Work out the finished part from the listing and answer in its coordinate system (mm). A direction names the side the tool comes from. Give positions to 0.01 mm unless a question says otherwise; leave off trailing zeros. Loops run counter-clockwise (first coordinate to the right, second up) from the corner with the lowest first, then second, coordinate; pieces in that order, holes last. Notation, with made-up numbers: (-8.5, -9.5) - (35.5, -9.5) arc R9 cw to (35.5, 4.5) - close; hole circle Ø1 at (67.25, 87). An arc over 180 degrees is marked (long way). Use one line per item in the form item = value. Start each with the question number.
Solid Edge part; units mm, degrees
sketch "Sketch1" plane through (0, 0, -1.75) normal (0, 0, 1) x (1, 0, 0)
  line L0 (-3.447, 1.4766) -> (7.158, 26.233)
  line L1 (2.2918, -2.9682) -> (23.6093, 13.4911)
  arc A0 (23.6093, 13.4911) -> (7.158, 26.233) centre (17.0395, 22) ccw
  arc A1 (2.2918, -2.9682) -> (-3.447, 1.4766) centre (0, 0) cw
sketch "Sketch2" plane through (17.0395, 0, 0) normal (-1, 0, 0) x (0, -1, 0)
  line L0 (-32.75, -0.3358) -> (-31.3358, -1.75)
  line L1 (-32.75, -3.1642) -> (-31.3358, -1.75)
  line L2 (-32.75, -3.1642) -> (-34.1642, -1.75)
  line L3 (-32.75, -0.3358) -> (-34.1642, -1.75)
sweep "Riemen_Twist" add profiles "Sketch2" path "Sketch1"
properties material "(None)"
1) Find the intervals of material crossed by probe 1 along X at (y, z) = (12, -3); probe 2 along Y at (x, z) = (13, -1.1); probe 3 along Y at (x, z) = (25.5, -1.65), in increasing order.
2) Determine the mould class of faces 4 (the conical face through (23.99, 30.52, -2.92)), 5 (the conical face through (-1.543, -2.07, -1.996)), 6 (the flat face through (13.227, 4.594, -2.467)) for opening direction Y: released by +Y, released by -Y, zero draft, split by the parting line, or undercut.
3) A cutting plane is placed at B-B (z = -2.5). Give the vertices of the cut face in (x, y), plus the area to 3 significant figures.
4) Flat-ended cylindrical pins translate along their axes: pin 1 Ø1 at (x, z) = (16.5, -2) entering from -Y; pin 2 Ø8 at (x, y) = (0.5, 13.5) entering from -Z; pin 3 Ø8 at (x, y) = (8.5, 0) entering from +Z; pin 4 Ø8 at (x, y) = (12.5, 15.5) entering from -Z. Find the tip coordinate at first contact, or state that the pin passes through.
5) A tool of negligible diameter and unlimited length cuts with its end or side. For faces 1 (the flat face through (12.38, 5.7, -1.03)), 2 (the flat face through (2.59, 13.75, -2.45)), 3 (the flat face through (13.24, 4.58, -1.05)), from which of +Z, -Z, +X, -X, +Y, -Y can it reach the whole face along a straight path? Write none if from no direction.
6) A cutting plane is placed at A-A (y = 22). Give the vertices of the cut face in (x, z).
Answer sheet:
q1.probe_1 = 0.88 to 1.24, 21.41 to 21.95
q1.probe_2 = 4.33 to 6.27, 31.13 to 32.78
q1.probe_3 = 13.4 to 17.82, 26.18 to 30.6
q2.face_4 = split by the parting line
q2.face_5 = undercut
q2.face_6 = released by -Y
q3.outline = (-4.06, 1.74) arc R4.41 ccw to (2.7, -3.49) - (24.02, 12.97) arc R11.41 ccw (long way) to (6.55, 26.49) - close; hole (-2.84, 1.22) arc R3.09 ccw to (1.89, -2.44) - (23.2, 14.02) arc R10.09 ccw (long way) to (7.77, 25.97) - close
q3.area = 137 mm²
q4.pin_1 = 5.88
q4.pin_2 = -3.16
q4.pin_3 = -0.34
q4.pin_4 = through
q5.face_1 = +Z
q5.face_2 = -Z
q5.face_3 = +Z, +X, -Y
q6.outline = (3.81, -1.75) - (5.34, -3.16) - (6.88, -1.75) - (5.34, -0.34) - close; (26.38, -1.75) - (27.79, -3.16) - (29.2, -1.75) - (27.79, -0.34) - close
